The figure shows three views and two pictorial views of one solid part (mm, origin at its lowest corner). Answer the questions. Coordinates: 2 decimals unless noted, no trailing zeros. Order: outer loops, then holes, each group sorted by start corner. A loop starts at its lowest first (then second) coordinate and runs counter-clockwise, first axis right, second up. Notation, with made-up numbers: (52, 38.5) -> (57, 38.5) arc R19 cw to (57, 72.5) -> close; hole circle Ø3 at (79.25, -3). An arc over 180 degrees is marked (long way). Write item = value, one per line. Start each with the question number.
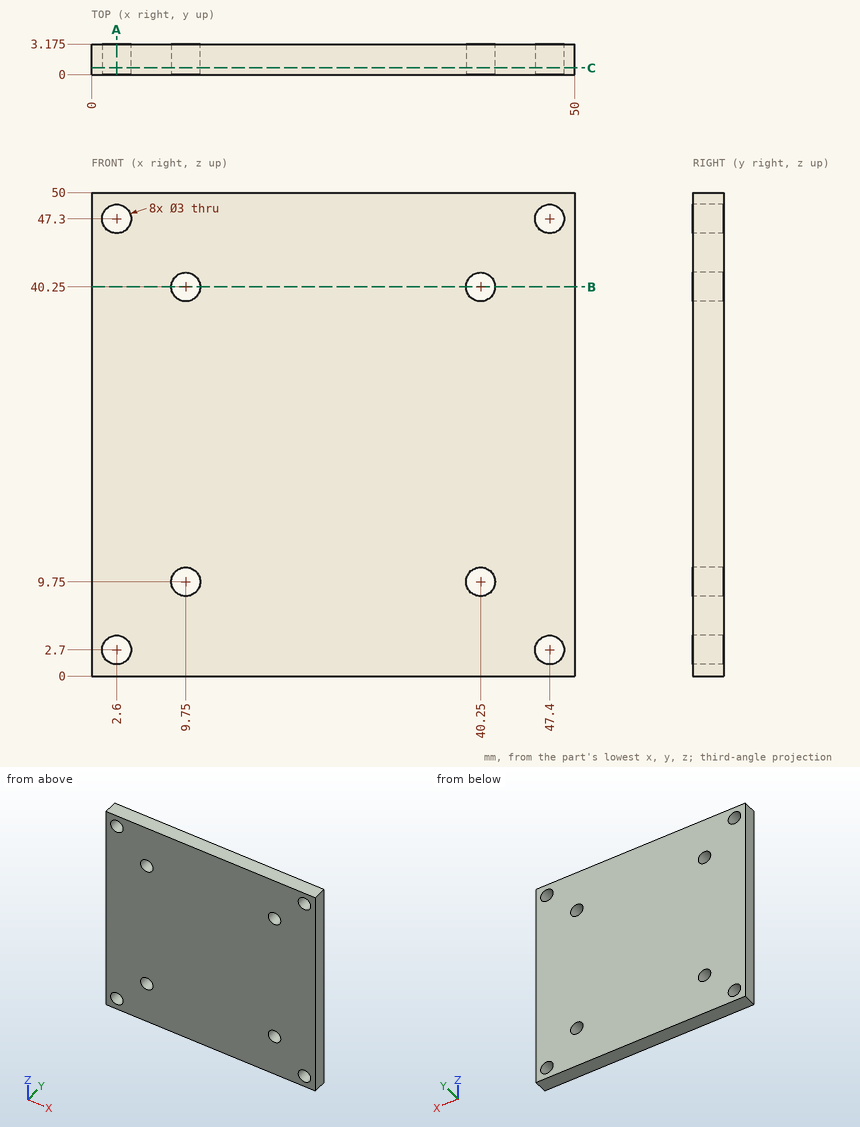
Item 1: Consider probe 1 along X at (y, z) = (2.25, 9.75); probe 2 along X at (y, z) = (1.8, 2.7); probe 3 along Z at (x, y) = (2.6, 2.05). Determine where each line is inside the solid, lowest interval first.
Item 2: Section A-A, the plane x = 2.6 is taken. Give the vertices of the cut face in (y, z) (3 decimals), then the cut area to 3 significant figures.
Item 3: Section B-B, the plane z = 40.25 is taken. Give the vertices of the cut face in (x, y) (3 decimals), then the cut area to 3 significant figures.
Item 4: Section C-C, the plane y = 0.7 is taken. Give the number of separate pieces and of enclosed holes in the cut face, then the cut area to 3 significant figures.
Item 5: This flat-tipped pin is pushed along its axis until it touches: pin 1 (2.5 mm diameter, centred on x = 47.4, z = 47.3, fed in from -Y). Where does it stop, or does it pass through?
A:
q1.probe_1 = 0 to 8.25, 11.25 to 38.75, 41.75 to 50
q1.probe_2 = 0 to 1.1, 4.1 to 45.9, 48.9 to 50
q1.probe_3 = 0 to 1.2, 4.2 to 45.8, 48.8 to 50
q2.outline = (0, 0) -> (3.175, 0) -> (3.175, 1.2) -> (0, 1.2) -> close; (0, 4.2) -> (3.175, 4.2) -> (3.175, 45.8) -> (0, 45.8) -> close; (0, 48.8) -> (3.175, 48.8) -> (3.175, 50) -> (0, 50) -> close
q2.area = 140 mm^2
q3.outline = (0, 0) -> (8.25, 0) -> (8.25, 3.175) -> (0, 3.175) -> close; (11.25, 0) -> (38.75, 0) -> (38.75, 3.175) -> (11.25, 3.175) -> close; (41.75, 0) -> (50, 0) -> (50, 3.175) -> (41.75, 3.175) -> close
q3.area = 140 mm^2
q4.separate_pieces = 1
q4.enclosed_holes = 8
q4.area = 2,440 mm^2
q5.pin_1 = through
